Model file for the job. Use its own axes, mm. A direction names the side the tool comes from. Coordinates: 2 decimals unless noted, no trailing zeros. Loops run counter-clockwise (first coordinate to the right, second up) from the corner with the lowest first, then second, coordinate; pieces in that order, holes last. Notation, with made-up numbers: M -9,-16.5 L -1,-16.5 A20 ccw -1,1.5 Z; hole C 10,7 d5. An arc over 180 degrees is marked long. Write item = value, one per line. Start each with the question number.
from build123d import *

# Parameters (mm, degrees)
SKETCH012_W    = 32
SKETCH012_H    = 120
PAD005_DEPTH   = 20.5
THICKNESS001_T = -1.5
SKETCH013_W    = 1.5
SKETCH013_H    = 20.5
PAD006_DEPTH   = 29
FILLET007_R    = 3
FILLET008_R    = 5


with BuildPart() as part:
    # Sketch012 → Pad005 (new body)
    with BuildSketch(Plane.XY):
        Rectangle(SKETCH012_W, SKETCH012_H)
    extrude(amount=PAD005_DEPTH)

    # Thickness001
    thickness001_openings = [part.faces().sort_by_distance(p)[0] for p in [
        (0, 0, 20.5),
    ]]
    offset(amount=THICKNESS001_T, openings=thickness001_openings)

    # Sketch013 (on DatumPlane) → Pad006 (join)
    with BuildSketch(Plane(origin=(-14.5, -20, 0), x_dir=(0, 1, 0), z_dir=(1, 0, 0))):
        with Locations((0, 10.25)):
            Rectangle(SKETCH013_W, SKETCH013_H)
    extrude(amount=PAD006_DEPTH)

    # Fillet007
    fillet007_edges = [part.edges().sort_by_distance(p)[0] for p in [
        (-14.5, 58.5, 11),
        (14.5, 58.5, 11),
        (16, 60, 10.25),
        (-16, 60, 10.25),
        (-14.5, -58.5, 11),
        (-16, -60, 10.25),
        (-14.5, -20.75, 11),
        (-14.5, -19.25, 11),
        (14.5, -19.25, 11),
        (14.5, -20.75, 11),
        (14.5, -58.5, 11),
        (16, -60, 10.25),
    ]]
    fillet(fillet007_edges, radius=FILLET007_R)

    # Fillet008
    fillet008_edges = [part.edges().sort_by_distance(p)[0] for p in [
        (0, 58.5, 1.5),
        (-13.62132, 57.62132, 1.5),
        (13.62132, 57.62132, 1.5),
        (-14.5, 19.625, 1.5),
        (14.5, 19.625, 1.5),
        (-13.62132, -18.37132, 1.5),
        (13.62132, -18.37132, 1.5),
        (0, -19.25, 1.5),
    ]]
    fillet(fillet008_edges, radius=FILLET008_R)


with BuildPart() as part_1:
    # Body004 placement: moved
    add(part.part.moved(Location((-22, 83, 14))))


with BuildPart() as part_2:
    # Body005 placement: moved
    add(part_1.part.moved(Location((32, 0, 0))))


solid = part_2.part
Item 1: Cut at A-A (z = 24.25). Give the cut face in (x, y), plus the area to 3 significant figures.
Item 2: 3-axis set-ups, long thin cutter, end or side, ignore diameter. For faces 1 (the flat face through (26, 82, 24)), 2 (the flat face through (10, 44, 15.5)): which of +Z, -Z, +X, -X, +Y, -Y reach the whole face in a straight line?
Item 3: Pull direction X, two halves, no side cores. Call faces 3 (the cylindrical face through (-3.64, 64.65, 27.6)), 4 (the cylindrical face through (25.1, 23.86, 24.39)), 5 (the flat face through (10, 82, 14)): +X half, -X half, draft (parallel to the pull), parting line (faces both ways), or undercut.
Item 4: Cut at B-B (x = 12.5). Give the cut face in (y, z), plus the area to 3 significant figures.
Item 5: Cut at D-D (y = 99). Give the cut face in (x, z).
Item 6: Cut at C-C (y = 53.5). Give the cut face in (x, z), plus the area to 3 significant figures.
Item 7: Pin check, flat tips, straight feed: pin 1 Ø12 at (x, y) = (7.5, 93.5) entering from +Z; pin 2 Ø2 at (x, y) = (21, 122.5) entering from +Z. Stop position of each tip, or through.
Item 8: Probe L1, parallel to Y at x = 21.5, z = 26.5; L2, parallel to X at y = 113, z = 25.5; L3, parallel to Y at x = 15, z = 17.25. List the from-to ranges inside material, lowest first.
Reported:
q1.outline = M -6,26 A3 ccw -3,23 L 23,23 A3 ccw 26,26 L 26,140 A3 ccw 23,143 L -3,143 A3 ccw -6,140 Z; hole M -4.5,27.5 A3 ccw -1.5,24.5 L 21.5,24.5 A3 ccw 24.5,27.5 L 24.5,59.25 A3 ccw 21.5,62.25 L -1.5,62.25 A3 ccw -4.5,59.25 Z; hole M -4.5,66.75 A3 ccw -1.5,63.75 L 21.5,63.75 A3 ccw 24.5,66.75 L 24.5,138.5 A3 ccw 21.5,141.5 L -1.5,141.5 A3 ccw -4.5,138.5 Z
q1.area = 498 mm^2
q2.face_1 = +Z, -Z, +X, +Y, -Y
q2.face_2 = +Z
q3.face_3 = undercut
q3.face_4 = +X half
q3.face_5 = draft
q4.outline = M 23,14 L 143,14 L 143,34.5 L 141.5,34.5 L 141.5,20.5 A5 cw 136.5,15.5 L 68.75,15.5 A5 cw 63.75,20.5 L 63.75,34.5 L 62.25,34.5 L 62.25,15.5 L 24.5,15.5 L 24.5,34.5 L 23,34.5 Z
q4.area = 276 mm^2
q5.outline = M -6,14 L 26,14 L 26,34.5 L 24.5,34.5 L 24.5,20.5 A5 cw 19.5,15.5 L 0.5,15.5 A5 cw -4.5,20.5 L -4.5,34.5 L -6,34.5 Z
q6.outline = M -6,14 L 26,14 L 26,34.5 L 24.5,34.5 L 24.5,15.5 L -4.5,15.5 L -4.5,34.5 L -6,34.5 Z
q6.area = 105 mm^2
q7.pin_1 = 15.5
q7.pin_2 = 16.17
q8.L1 = 23 to 24.5, 62.25 to 63.75, 141.5 to 143
q8.L2 = -6 to -4.5, 24.5 to 26
q8.L3 = 23 to 24.5, 62.25 to 64.95, 140.3 to 143
